Here's how the part is built. I have some questions about the finished solid (model axes, mm). Coordinates: 2 decimals unless noted, no trailing zeros. Loops run counter-clockwise (first coordinate to the right, second up) from the corner with the lowest first, then second, coordinate; pieces in that order, holes last. Notation, with made-up numbers: (-38.75, -4) -> (-11.75, -4) arc R28 cw to (-11.75, 30) -> close; hole circle Ø7 at (-29, -7). An arc over 180 degrees is marked (long way). Answer as a JSON object with one key per item and string values. Group by question number.
Q1. I'm going to push a flat-ended pin straight in: pin 1 (2.5 mm diameter, centred on x = 24, z = 18, fed in from -Y) (3 decimals). Where does the tip first touch, or does it pass through?
Q2. I want a section at B-B on y = 3.4. Count the separate pieces of the cut face and the enclosed holes in it, then the cut area to 3 significant figures.
Q3. I want a section at C-C on z = 35.5. Write out the boundary of the cut face in (x, y), then the cut area to 3 significant figures.
Q4. I want a section at A-A on x = 24. Write out the boundary of the cut face in (y, z), then the cut area to 3 significant figures.
Q5. I need wall thicknesses on line 1 (X direction, y = 2.4, z = 20); line 2 (X direction, y = 1, z = 18); line 3 (Z direction, x = 36, y = 2.5). Which ranges of each line are inside material? Lowest first, please.
```python
from build123d import *

# Parameters (mm, degrees)
SKETCH_1_W          = 110
SKETCH_1_H          = 85
SKETCH_1_R          = 1.7
EXTRUDE_1_DEPTH     = 4
SKETCH_2_R          = 1.7
CUT_EXTRUDE_1_DEPTH = 10
FILLET_1_R          = 10


with BuildPart() as part:
    # 草图1 → 凸台-拉伸1 (new body)
    with BuildSketch(Plane(origin=(0, 0, 0), x_dir=(1, 0, 0), z_dir=(0, 1, 0))):
        Rectangle(SKETCH_1_W, SKETCH_1_H)
        with Locations(Location((24, 18, 0), (0, 0, 270))):
            Circle(SKETCH_1_R, mode=Mode.SUBTRACT)
        with Locations(Location((-24, 18, 0), (0, 0, 270))):
            Circle(SKETCH_1_R, mode=Mode.SUBTRACT)
        with Locations(Location((-24, -18, 0), (0, 0, 270))):
            Circle(SKETCH_1_R, mode=Mode.SUBTRACT)
        with Locations(Location((24, -18, 0), (0, 0, 270))):
            Circle(SKETCH_1_R, mode=Mode.SUBTRACT)
        with Locations(Location((-35.355, 35.355, 0), (0, 0, 270))):
            Circle(SKETCH_1_R, mode=Mode.SUBTRACT)
        with Locations(Location((35.355, 35.355, 0), (0, 0, 270))):
            Circle(SKETCH_1_R, mode=Mode.SUBTRACT)
        with Locations(Location((35.355, -35.355, 0), (0, 0, 270))):
            Circle(SKETCH_1_R, mode=Mode.SUBTRACT)
        with Locations(Location((-35.355, -35.355, 0), (0, 0, 270))):
            Circle(SKETCH_1_R, mode=Mode.SUBTRACT)
    extrude(amount=EXTRUDE_1_DEPTH)

    # 草图2 → 切除-拉伸1 (cut)
    with BuildSketch(Plane(origin=(0, 4, 0), x_dir=(1, 0, 0), z_dir=(0, 1, 0))):
        with Locations(Location((50, 20, 0), (0, 0, 270))):
            Circle(SKETCH_2_R)
        with Locations(Location((50, -20, 0), (0, 0, 270))):
            Circle(SKETCH_2_R)
        with Locations(Location((-50, 20, 0), (0, 0, 270))):
            Circle(SKETCH_2_R)
        with Locations(Location((-50, -20, 0), (0, 0, 270))):
            Circle(SKETCH_2_R)
    extrude(amount=-CUT_EXTRUDE_1_DEPTH, mode=Mode.SUBTRACT)

    # 圆角1
    fillet_1_edges = [part.edges().sort_by_distance(p)[0] for p in [
        (55, 2, 42.5),
        (-55, 2, 42.5),
        (-55, 2, -42.5),
        (55, 2, -42.5),
    ]]
    fillet(fillet_1_edges, radius=FILLET_1_R)


solid = part.part
```
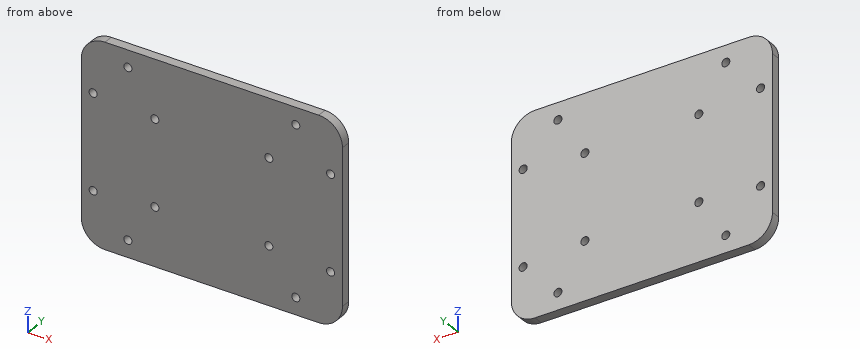
Result set:
{
 "1": {"pin 1": "passes through"},
 "2": {"separate pieces": "1", "enclosed holes": "12", "area": "9,160 mm²"},
 "3": {"outline": "(-54.54, 0) -> (-37.05, 0) -> (-37.05, 4) -> (-54.54, 4) -> close; (-33.66, 0) -> (33.66, 0) -> (33.66, 4) -> (-33.66, 4) -> close; (37.05, 0) -> (54.54, 0) -> (54.54, 4) -> (37.05, 4) -> close", "area": "409 mm²"},
 "4": {"outline": "(0, -42.5) -> (4, -42.5) -> (4, -19.7) -> (0, -19.7) -> close; (0, -16.3) -> (4, -16.3) -> (4, 16.3) -> (0, 16.3) -> close; (0, 19.7) -> (4, 19.7) -> (4, 42.5) -> (0, 42.5) -> close", "area": "313 mm²"},
 "5": {"line 1": "x = -55 to -51.7, -48.3 to 48.3, 51.7 to 55", "line 2": "x = -55 to -25.7, -22.3 to 22.3, 25.7 to 55", "line 3": "z = -42.5 to -36.93, -33.78 to 33.78, 36.93 to 42.5"}
}
